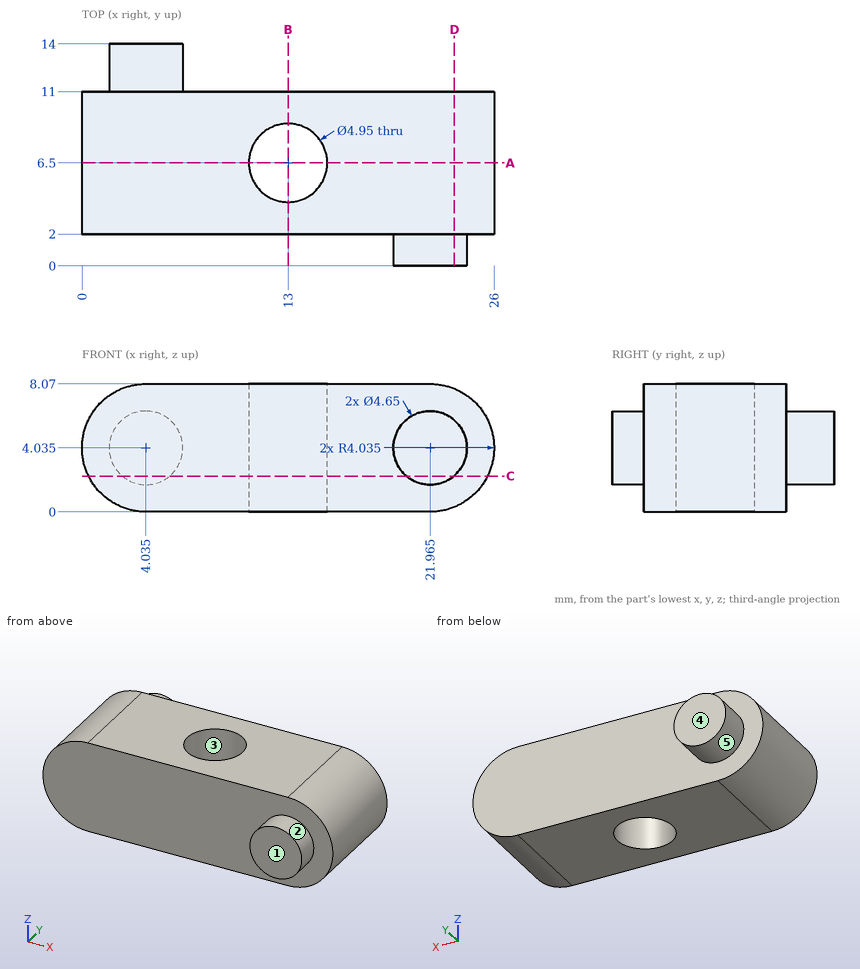
Geometry: see drawing. Coordinates: mm, zero at the bounding-box minimum. A direction names the side the tool comes from. Round coordinates to 2 decimals unless told otherwise and drop trailing zeros. Loops run counter-clockwise (first coordinate to the right, second up) from the corner with the lowest first, then second, coordinate; pieces in that order, holes last. Notation, with made-up numbers: (-13, -11.5) -> (21, -11.5) arc R4 cw to (21, -7.5) -> close; hole circle Ø8 at (80.25, 2.5). An arc over 180 degrees is marked (long way). Use one line per item in the form item = value. Start each with the question number.
Item 1: Material intervals for L1, parallel to Y at x = 13, z = 5.5 (3 decimals); L2, parallel to Y at x = 2.5, z = 1; L3, parallel to Y at x = 4.75, z = 5.25, sorted ascending. Write a range as from..to.
Item 2: Mould query, pull axis Y, two halves, no side actions, for the marked faces 1, 2 and 3. Classes: pulls with the +Y half, pulls with the -Y half, needs draft (parallel to the pull), parting line crosses it, or undercut.
Item 3: Set-up query: the marked faces 4 and 5. Return all of +Z, -Z, +X, -X, +Y, -Y with unobstructed straight access to the full face (end or side cutting, diameter ignored); none if empty.
Item 4: Section query B-B on x = 13. Return the cut outline in (y, z) (3 decimals), then the cut area to 3 significant figures.
Item 5: Section query A-A on y = 6.5. Return the cut outline in (x, z) (3 decimals), then the cut area to 3 significant figures.
Item 6: Contact query for flat-ended pins moving along their axis: pin 1 Ø4.5 at (x, y) = (13, 6.5) entering from -Z; pin 2 Ø1 at (y, z) = (8, 5.5) entering from -X; pin 3 Ø1 at (x, z) = (3.5, 4.5) entering from -Y; pin 4 Ø2.5 at (x, z) = (8.5, 3) entering from +Y. Output: stop coordinate, or through.
Item 7: Section query C-C on z = 2.25. Return the cut outline in (x, y) (3 decimals), then the cut area to 3 significant figures.
Item 8: Section query D-D on x = 23.5. Return the cut outline in (y, z).
Ans:
q1.L1 = 2..4.025, 8.975..11
q1.L2 = 2..11
q1.L3 = 2..14
q2.face_1 = pulls with the -Y half
q2.face_2 = needs draft
q2.face_3 = undercut
q3.face_4 = +Z, -Z, +X, -X, +Y
q3.face_5 = +Y
q4.outline = (2, 0) -> (4.025, 0) -> (4.025, 8.07) -> (2, 8.07) -> close; (8.975, 0) -> (11, 0) -> (11, 8.07) -> (8.975, 8.07) -> close
q4.area = 32.7 mm^2
q5.outline = (4.035, 0) -> (10.525, 0) -> (10.525, 8.07) -> (4.035, 8.07) arc R4.035 ccw to start; (15.475, 0) -> (21.965, 0) arc R4.035 ccw to (21.965, 8.07) -> (15.475, 8.07) -> close
q5.area = 156 mm^2
q6.pin_1 = through
q6.pin_2 = 0.12
q6.pin_3 = 2
q6.pin_4 = 11
q7.outline = (0.416, 2) -> (20.475, 2) -> (20.475, 0) -> (23.455, 0) -> (23.455, 2) -> (25.584, 2) -> (25.584, 11) -> (5.525, 11) -> (5.525, 14) -> (2.545, 14) -> (2.545, 11) -> (0.416, 11) -> close; hole circle Ø4.95 at (13, 6.5)
q7.area = 222 mm^2
q8.outline = (0, 2.29) -> (2, 2.29) -> (2, 0.3) -> (11, 0.3) -> (11, 7.77) -> (2, 7.77) -> (2, 5.78) -> (0, 5.78) -> close
